```python
from build123d import *

# Parameters (mm, degrees)
F0_W         = 50.8
F0_H         = 50.8
F1_DEPTH     = 25.4
F2_DEPTH     = 25.4
F3_R         = 12.7
F4_R         = 12.7
F5_T1_DEPTH  = 25.4
F5_S5_W      = 12.7
F5_S5_H      = 12.7
F5_T6_DEPTH  = 12.7
F5_S11_W     = 12.7
F5_S11_H     = 12.7
F5_T12_DEPTH = 12.7
F5_S17_W     = 12.7
F5_S17_H     = 12.7
F5_T18_DEPTH = 12.7
F5_S23_W     = 12.7
F5_S23_H     = 12.7
F5_T24_DEPTH = 12.7
F5_S29_W     = 12.7
F5_S29_H     = 12.7
F5_T30_DEPTH = 12.7
F5_S35_W     = 12.7
F5_S35_H     = 12.7
F5_T36_DEPTH = 12.7
F5_S41_W     = 12.7
F5_S41_H     = 12.7
F5_T42_DEPTH = 12.7
F5_S47_W     = 12.7
F5_S47_H     = 12.7
F5_T48_DEPTH = 12.7


# Not quite as in the source:
# - a fillet or chamfer that OpenCascade refuses, or shapes differently, is made with other operations: its cross-section is extruded or revolved along the edge and cut away or added


with BuildPart() as f1:
    # F0 (on Top) → F1 (new body)
    with BuildSketch(Plane.XY):
        with Locations((-3.5267624348, -4.2439938247)):
            Rectangle(F0_W, F0_H)
    extrude(amount=F1_DEPTH)

    # F2 (add): a face of the model
    f2_faces = [f1.faces().sort_by_distance(p)[0] for p in [
        (-3.5267624348, -4.2439938247, 0),
    ]]
    extrude(f2_faces, amount=F2_DEPTH)

    # F3
    f3_edges = [f1.edges().sort_by_distance(p)[0] for p in [
        (-3.526762, -29.643994, 25.4),
        (-28.926762, -4.243994, 25.4),
        (-3.526762, 21.156006, 25.4),
        (21.873238, -4.243994, 25.4),
    ]]
    fillet(f3_edges, radius=F3_R)

    # F4
    f4_edges = [f1.edges().sort_by_distance(p)[0] for p in [
        (-3.526762, -29.643994, -25.4),
        (-28.926762, -4.243994, -25.4),
        (-3.526762, 21.156006, -25.4),
        (21.873238, -4.243994, -25.4),
    ]]
    fillet(f4_edges, radius=F4_R)

    # F5: fillet of radius 12.7 on 4 edges, made by hand

    # F5_s2 → F5_t1 (cut)
    with BuildSketch(Plane.XY.offset(-12.7)):
        with BuildLine():
            ThreePointArc((-28.9267624348, -16.9439938247), (-25.2070185559, -25.9242499458), (-16.2267624348, -29.6439938247))
            Line((-16.2267624348, -29.6439938247), (-28.9267624348, -29.6439938247))
            Line((-28.9267624348, -29.6439938247), (-28.9267624348, -16.9439938247))
        make_face()
        with BuildLine():
            ThreePointArc((-16.2267624348, 21.1560061753), (-25.2070185559, 17.4362622963), (-28.9267624348, 8.4560061753))
            Line((-28.9267624348, 8.4560061753), (-28.9267624348, 21.1560061753))
            Line((-28.9267624348, 21.1560061753), (-16.2267624348, 21.1560061753))
        make_face()
        with BuildLine():
            ThreePointArc((9.1732375652, 21.1560061753), (18.1534936862, 17.4362622963), (21.8732375652, 8.4560061753))
            Line((21.8732375652, 8.4560061753), (21.8732375652, 21.1560061753))
            Line((21.8732375652, 21.1560061753), (9.1732375652, 21.1560061753))
        make_face()
        with BuildLine():
            ThreePointArc((21.8732375652, -16.9439938247), (18.1534936862, -25.9242499458), (9.1732375652, -29.6439938247))
            Line((9.1732375652, -29.6439938247), (21.8732375652, -29.6439938247))
            Line((21.8732375652, -29.6439938247), (21.8732375652, -16.9439938247))
        make_face()
    extrude(amount=F5_T1_DEPTH, mode=Mode.SUBTRACT)


with BuildPart() as f5_tool4:
    # F5_s5 → F5_t6 (new body)
    with BuildSketch(Plane.YZ.offset(9.1732375652)):
        with Locations((-23.2939938247, 19.05)):
            Rectangle(F5_S5_W, F5_S5_H)
    extrude(amount=F5_T6_DEPTH)

    # F5_s7 → F5_t8 (revolve, cut)
    with BuildSketch(Plane(origin=(9.1732375652, -16.9439938247, 12.7), x_dir=(0, 0.7071067812, -0.7071067812), z_dir=(0, -0.7071067812, -0.7071067812))):
        with BuildLine():
            ThreePointArc((0, -12.7), (12.7, 0), (0, 12.7))
            Line((0, 12.7), (0, -12.7))
        make_face()
    revolve(axis=Axis((9.1732375652, -16.9439938247, 12.7), (1, 0, 0)), mode=Mode.SUBTRACT)


with BuildPart() as f1_1:
    add(f1.part)

    # F5_t3: cut F5_tool4
    add(f5_tool4.part, mode=Mode.SUBTRACT)


with BuildPart() as f5_tool10:
    # F5_s11 → F5_t12 (new body)
    with BuildSketch(Plane.YZ.offset(9.1732375652)):
        with Locations((-23.2939938247, -19.05)):
            Rectangle(F5_S11_W, F5_S11_H)
    extrude(amount=F5_T12_DEPTH)

    # F5_s13 → F5_t14 (revolve, cut)
    with BuildSketch(Plane(origin=(9.1732375652, -16.9439938247, -12.7), x_dir=(0, 0.7071067812, 0.7071067812), z_dir=(0, 0.7071067812, -0.7071067812))):
        with BuildLine():
            ThreePointArc((0, -12.7), (12.7, 0), (0, 12.7))
            Line((0, 12.7), (0, -12.7))
        make_face()
    revolve(axis=Axis((9.1732375652, -16.9439938247, -12.7), (1, 0, 0)), mode=Mode.SUBTRACT)


with BuildPart() as f1_2:
    add(f1_1.part)

    # F5_t9: cut F5_tool10
    add(f5_tool10.part, mode=Mode.SUBTRACT)


with BuildPart() as f5_tool16:
    # F5_s17 → F5_t18 (new body)
    with BuildSketch(Plane.XZ.offset(-8.4560061753)):
        with Locations((15.5232375652, 19.05)):
            Rectangle(F5_S17_W, F5_S17_H)
    extrude(amount=-F5_T18_DEPTH)

    # F5_s19 → F5_t20 (revolve, cut)
    with BuildSketch(Plane(origin=(9.1732375652, 8.4560061753, 12.7), x_dir=(-0.7071067812, 0, -0.7071067812), z_dir=(0.7071067812, 0, -0.7071067812))):
        with BuildLine():
            ThreePointArc((0, -12.7), (12.7, 0), (0, 12.7))
            Line((0, 12.7), (0, -12.7))
        make_face()
    revolve(axis=Axis((9.1732375652, 8.4560061753, 12.7), (0, 1, 0)), mode=Mode.SUBTRACT)


with BuildPart() as f1_3:
    add(f1_2.part)

    # F5_t15: cut F5_tool16
    add(f5_tool16.part, mode=Mode.SUBTRACT)


with BuildPart() as f5_tool22:
    # F5_s23 → F5_t24 (new body)
    with BuildSketch(Plane.XZ.offset(-8.4560061753)):
        with Locations((15.5232375652, -19.05)):
            Rectangle(F5_S23_W, F5_S23_H)
    extrude(amount=-F5_T24_DEPTH)

    # F5_s25 → F5_t26 (revolve, cut)
    with BuildSketch(Plane(origin=(9.1732375652, 8.4560061753, -12.7), x_dir=(-0.7071067812, 0, 0.7071067812), z_dir=(-0.7071067812, 0, -0.7071067812))):
        with BuildLine():
            ThreePointArc((0, -12.7), (12.7, 0), (0, 12.7))
            Line((0, 12.7), (0, -12.7))
        make_face()
    revolve(axis=Axis((9.1732375652, 8.4560061753, -12.7), (0, 1, 0)), mode=Mode.SUBTRACT)


with BuildPart() as f1_4:
    add(f1_3.part)

    # F5_t21: cut F5_tool22
    add(f5_tool22.part, mode=Mode.SUBTRACT)


with BuildPart() as f5_tool28:
    # F5_s29 → F5_t30 (new body)
    with BuildSketch(Plane.XZ.offset(-8.4560061753)):
        with Locations((-22.5767624348, -19.05)):
            Rectangle(F5_S29_W, F5_S29_H)
    extrude(amount=-F5_T30_DEPTH)

    # F5_s31 → F5_t32 (revolve, cut)
    with BuildSketch(Plane(origin=(-16.2267624348, 8.4560061753, -12.7), x_dir=(0.7071067812, 0, 0.7071067812), z_dir=(-0.7071067812, 0, 0.7071067812))):
        with BuildLine():
            ThreePointArc((0, -12.7), (12.7, 0), (0, 12.7))
            Line((0, 12.7), (0, -12.7))
        make_face()
    revolve(axis=Axis((-16.2267624348, 8.4560061753, -12.7), (0, 1, 0)), mode=Mode.SUBTRACT)


with BuildPart() as f1_5:
    add(f1_4.part)

    # F5_t27: cut F5_tool28
    add(f5_tool28.part, mode=Mode.SUBTRACT)


with BuildPart() as f5_tool34:
    # F5_s35 → F5_t36 (new body)
    with BuildSketch(Plane.XZ.offset(-8.4560061753)):
        with Locations((-22.5767624348, 19.05)):
            Rectangle(F5_S35_W, F5_S35_H)
    extrude(amount=-F5_T36_DEPTH)

    # F5_s37 → F5_t38 (revolve, cut)
    with BuildSketch(Plane(origin=(-16.2267624348, 8.4560061753, 12.7), x_dir=(0.7071067812, 0, -0.7071067812), z_dir=(0.7071067812, 0, 0.7071067812))):
        with BuildLine():
            ThreePointArc((0, -12.7), (12.7, 0), (0, 12.7))
            Line((0, 12.7), (0, -12.7))
        make_face()
    revolve(axis=Axis((-16.2267624348, 8.4560061753, 12.7), (0, 1, 0)), mode=Mode.SUBTRACT)


with BuildPart() as f1_6:
    add(f1_5.part)

    # F5_t33: cut F5_tool34
    add(f5_tool34.part, mode=Mode.SUBTRACT)


with BuildPart() as f5_tool40:
    # F5_s41 → F5_t42 (new body)
    with BuildSketch(Plane.YZ.offset(-16.2267624348)):
        with Locations((-23.2939938247, -19.05)):
            Rectangle(F5_S41_W, F5_S41_H)
    extrude(amount=-F5_T42_DEPTH)

    # F5_s43 → F5_t44 (revolve, cut)
    with BuildSketch(Plane(origin=(-16.2267624348, -16.9439938247, -12.7), x_dir=(0, 0.7071067812, 0.7071067812), z_dir=(0, -0.7071067812, 0.7071067812))):
        with BuildLine():
            ThreePointArc((0, -12.7), (12.7, 0), (0, 12.7))
            Line((0, 12.7), (0, -12.7))
        make_face()
    revolve(axis=Axis((-16.2267624348, -16.9439938247, -12.7), (-1, 0, 0)), mode=Mode.SUBTRACT)


with BuildPart() as f1_7:
    add(f1_6.part)

    # F5_t39: cut F5_tool40
    add(f5_tool40.part, mode=Mode.SUBTRACT)


with BuildPart() as f5_tool46:
    # F5_s47 → F5_t48 (new body)
    with BuildSketch(Plane.YZ.offset(-16.2267624348)):
        with Locations((-23.2939938247, 19.05)):
            Rectangle(F5_S47_W, F5_S47_H)
    extrude(amount=-F5_T48_DEPTH)

    # F5_s49 → F5_t50 (revolve, cut)
    with BuildSketch(Plane(origin=(-16.2267624348, -16.9439938247, 12.7), x_dir=(0, 0.7071067812, -0.7071067812), z_dir=(0, 0.7071067812, 0.7071067812))):
        with BuildLine():
            ThreePointArc((0, -12.7), (12.7, 0), (0, 12.7))
            Line((0, 12.7), (0, -12.7))
        make_face()
    revolve(axis=Axis((-16.2267624348, -16.9439938247, 12.7), (-1, 0, 0)), mode=Mode.SUBTRACT)


with BuildPart() as f1_8:
    add(f1_7.part)

    # F5_t45: cut F5_tool46
    add(f5_tool46.part, mode=Mode.SUBTRACT)


solid = f1_8.part
```
Work out the finished part from the listing and answer in its coordinate system (mm). Coordinates: 2 decimals unless noted, no trailing zeros. Loops run counter-clockwise (first coordinate to the right, second up) from the corner with the lowest first, then second, coordinate; pieces in that order, holes last.
1) Consider probe 1 along X at (y, z) = (-17.5, 0); probe 2 along X at (y, z) = (-25, -5); probe 3 along Y at (x, z) = (11, -1). Determine where each line is inside the solid, lowest interval first.
Results:
probe 1: x = -28.91 to 21.86
probe 2: x = -26.04 to 18.99
probe 3: y = -29.51 to 21.02
2) Flat-ended cylindrical pins translate along their axes: pin 1 (8 mm diameter, centred on x = 13.5, y = -2, fed in from +Z); pin 2 (8 mm diameter, centred on x = 4.5, z = -17, fed in from -Y); pin 3 (10 mm diameter, centred on x = 14.5, z = 6.5, fed in from +Y). Find the tip coordinate at first contact, or state that the pin passes through.
Results:
pin 1: stops at z = 25.4
pin 2: stops at y = -29.64
pin 3: stops at y = 21.15
3) For a pull along Y with two mould halves and no side action, classify faces 1 (the cylindrical face through (-25.31, -25.82, -0.18)), 2 (the flat face through (-4, -4, 25.4)), 3 (the flat face through (-4, 21.156, 0)) as +Y half, -Y half, draft (parallel to the pull), parting line (faces both ways), or undercut.
Results:
face 1: -Y half
face 2: draft
face 3: +Y half
4) Section B-B (z = 10) is taken. Give the vertices of the cut face in (x, y).
Results:
outline: (-28.93, -16.94) arc R12.7 ccw to (-16.23, -29.64) - (9.17, -29.64) arc R12.7 ccw to (21.87, -16.94) - (21.87, 8.46) arc R12.7 ccw to (9.17, 21.16) - (-16.23, 21.16) arc R12.7 ccw to (-28.93, 8.46) - close
5) Section A-A (y = -16) is taken. Give the vertices of the cut face in (x, z), plus the area to 3 significant figures.
Results:
outline: (-28.93, -12.7) arc R12.7 ccw to (-16.23, -25.4) - (9.17, -25.4) arc R12.7 ccw to (21.87, -12.7) - (21.87, 12.7) arc R12.7 ccw to (9.17, 25.4) - (-16.23, 25.4) arc R12.7 ccw to (-28.93, 12.7) - close
area: 2,440 mm2
